```python
from build123d import *

# Parameters (mm, degrees)
BOSS_EXTRUDE1_DEPTH                     = 24
FILLET1_R                               = 1.5
SHELL1_T                                = -2
BOSS_EXTRUDE2_DEPTH                     = 6.2
CUT_EXTRUDE1_DEPTH                      = 5
FILLET2_R                               = 0.8
BOSS_EXTRUDE4_START                     = -1
SKETCH4_R                               = 5
BOSS_EXTRUDE4_DEPTH                     = 23
CBORE_FOR_M5_HEX_HEAD_BOLT1_D           = 3.7
CBORE_FOR_M5_HEX_HEAD_BOLT1_CBORE_D     = 7.5
CBORE_FOR_M5_HEX_HEAD_BOLT1_CBORE_DEPTH = 12


with BuildPart() as part:
    # Sketch1 → Boss-Extrude1 (new body)
    with BuildSketch(Plane(origin=(0, 0, 0), x_dir=(1, 0, 0), z_dir=(0, 1, 0))):
        with BuildLine():
            Line((74.5, -51.5), (74.5, 51.5))
            ThreePointArc((74.5, 51.5), (73.621320344, 53.621320344), (71.5, 54.5))
            Line((71.5, 54.5), (-71.5, 54.5))
            ThreePointArc((-71.5, 54.5), (-73.621320344, 53.621320344), (-74.5, 51.5))
            Line((-74.5, 51.5), (-74.5, -51.5))
            ThreePointArc((-74.5, -51.5), (-73.621320344, -53.621320344), (-71.5, -54.5))
            Line((-71.5, -54.5), (71.5, -54.5))
            ThreePointArc((71.5, -54.5), (73.621320344, -53.621320344), (74.5, -51.5))
        make_face()
    extrude(amount=BOSS_EXTRUDE1_DEPTH)

    # Fillet1
    fillet1_edges = [part.edges().sort_by_distance(p)[0] for p in [
        (-73.621320344, 24, -53.621320344),
        (-74.5, 24, 0),
        (-73.621320344, 24, 53.621320344),
        (0, 24, 54.5),
        (73.621320344, 24, 53.621320344),
        (74.5, 24, 0),
        (73.621320344, 24, -53.621320344),
        (0, 24, -54.5),
    ]]
    fillet(fillet1_edges, radius=FILLET1_R)

    # Shell1
    shell1_openings = [part.faces().sort_by_distance(p)[0] for p in [
        (0, 0, 0),
    ]]
    offset(amount=SHELL1_T, openings=shell1_openings, kind=Kind.INTERSECTION)

    # Sketch2 → Boss-Extrude2 (add)
    with BuildSketch(Plane(origin=(0, 0, 0), x_dir=(1, 0, 0), z_dir=(0, 1, 0))):
        with BuildLine():
            Line((-78, 51.5), (-78, -51.5))
            ThreePointArc((-78, -51.5), (-76.096194078, -56.096194078), (-71.5, -58))
            Line((-71.5, -58), (71.5, -58))
            ThreePointArc((71.5, -58), (76.096194078, -56.096194078), (78, -51.5))
            Line((78, -51.5), (78, 51.5))
            ThreePointArc((78, 51.5), (76.096194078, 56.096194078), (71.5, 58))
            Line((71.5, 58), (-71.5, 58))
            ThreePointArc((-71.5, 58), (-76.096194078, 56.096194078), (-78, 51.5))
        make_face()
        with BuildLine():
            Line((72.5, -51.5), (72.5, 51.5))
            ThreePointArc((72.5, 51.5), (72.207106781, 52.207106781), (71.5, 52.5))
            Line((71.5, 52.5), (-71.5, 52.5))
            ThreePointArc((-71.5, 52.5), (-72.207106781, 52.207106781), (-72.5, 51.5))
            Line((-72.5, 51.5), (-72.5, -51.5))
            ThreePointArc((-72.5, -51.5), (-72.207106781, -52.207106781), (-71.5, -52.5))
            Line((-71.5, -52.5), (71.5, -52.5))
            ThreePointArc((71.5, -52.5), (72.207106781, -52.207106781), (72.5, -51.5))
        make_face(mode=Mode.SUBTRACT)
    extrude(amount=BOSS_EXTRUDE2_DEPTH)

    # Sketch3 → Cut-Extrude1 (cut)
    with BuildSketch(Plane.XZ):
        with BuildLine():
            Line((-71.5, -56.5), (71.5, -56.5))
            ThreePointArc((71.5, -56.5), (75.035533906, -55.035533906), (76.5, -51.5))
            Line((76.5, -51.5), (76.5, 51.5))
            ThreePointArc((76.5, 51.5), (75.035533906, 55.035533906), (71.5, 56.5))
            Line((71.5, 56.5), (-71.5, 56.5))
            ThreePointArc((-71.5, 56.5), (-75.035533906, 55.035533906), (-76.5, 51.5))
            Line((-76.5, 51.5), (-76.5, -51.5))
            ThreePointArc((-76.5, -51.5), (-75.035533906, -55.035533906), (-71.5, -56.5))
        make_face()
        with BuildLine():
            Line((74, -51.5), (74, 51.5))
            ThreePointArc((74, 51.5), (73.267766953, 53.267766953), (71.5, 54))
            Line((71.5, 54), (-71.5, 54))
            ThreePointArc((-71.5, 54), (-73.267766953, 53.267766953), (-74, 51.5))
            Line((-74, 51.5), (-74, -51.5))
            ThreePointArc((-74, -51.5), (-73.267766953, -53.267766953), (-71.5, -54))
            Line((-71.5, -54), (71.5, -54))
            ThreePointArc((71.5, -54), (73.267766953, -53.267766953), (74, -51.5))
        make_face(mode=Mode.SUBTRACT)
    extrude(amount=-CUT_EXTRUDE1_DEPTH, mode=Mode.SUBTRACT)

    # Fillet2
    fillet2_edges = [part.edges().sort_by_distance(p)[0] for p in [
        (-76.096194078, 6.2, -56.096194078),
        (-78, 6.2, 0),
        (-76.096194078, 6.2, 56.096194078),
        (0, 6.2, 58),
        (76.096194078, 6.2, 56.096194078),
        (78, 6.2, 0),
        (76.096194078, 6.2, -56.096194078),
        (0, 6.2, -58),
        (74.5, 6.2, 0),
        (73.621320344, 6.2, -53.621320344),
        (0, 6.2, -54.5),
        (-73.621320344, 6.2, -53.621320344),
        (-74.5, 6.2, 0),
        (-73.621320344, 6.2, 53.621320344),
        (0, 6.2, 54.5),
        (73.621320344, 6.2, 53.621320344),
    ]]
    fillet(fillet2_edges, radius=FILLET2_R)

    # Sketch4 → Boss-Extrude4 (add)
    with BuildSketch(Plane(origin=(0, 24, 0), x_dir=(1, 0, 0), z_dir=(0, 1, 0)).offset(BOSS_EXTRUDE4_START)):
        with Locations((69, 49)):
            Circle(SKETCH4_R)
        with Locations((69, -49)):
            Circle(SKETCH4_R)
        with Locations((-69, 49)):
            Circle(SKETCH4_R)
        with Locations((-69, -49)):
            Circle(SKETCH4_R)
    extrude(amount=-BOSS_EXTRUDE4_DEPTH)

    # CBORE for M5 Hex Head Bolt1 (through all)
    with Locations(Plane(origin=(0, 24, 0), x_dir=(1, 0, 0), z_dir=(0, 1, 0))):
        with Locations((-69, -49), (69, -49), (-69, 49), (69, 49)):
            CounterBoreHole(CBORE_FOR_M5_HEX_HEAD_BOLT1_D / 2, CBORE_FOR_M5_HEX_HEAD_BOLT1_CBORE_D / 2, CBORE_FOR_M5_HEX_HEAD_BOLT1_CBORE_DEPTH)


solid = part.part
```
Geometry: final body of the model. Coordinates: model frame, mm. A direction names the side the tool comes from. Round coordinates to 2 decimals unless told otherwise and drop trailing zeros. Write each loop counter-clockwise with the first axis right and the second up, starting at its lowest first coordinate (ties: lowest second). Pieces come first, ordered by that corner, then holes. Notation, with made-up numbers: M -39,-2 L -17,-2 A5 ccw -17,2 Z; hole C 64,40.25 d10. An arc over 180 degrees is marked long. Answer in a Markdown table with one row per item. Add a question column.
(1) Draft query along X for faces 1 (the face through (-1, 15, 54.5)), 2 (the face through (72.464, 18.084, 50.436)). Return one class per face: pulls with the +X half, pulls with the -X half, needs draft (parallel to the pull), parting line crosses it, or undercut.
(2) Cut plane A-A, the plane y = 18.25. Return the cut outline in (x, z), then the cut area to 3 significant figures.
(3) Cut plane D-D, the plane z = -49. Give the number of separate pieces and of enclosed holes in the cut face, then the cut area to 3 significant figures.
(4) Cut plane C-C, the plane x = 61.5. Return the cut outline in (y, z), then the cut area to 3 significant figures.
(5) Reachability of faces 3 (the face through (-76.5, 2, 1)), 4 (the face through (70.468, 5.916, -47.874)), 5 (the face through (-65.536, 18.084, -47.564)) from +Z, -Z, +X, -X, +Y, -Y: full face, straight path, thin tool, end or side. Return the list, or none.
(6) Contact query for flat-ended pins moving along their axis: pin 1 (3 mm diameter, centred on y = 11.5, z = 29.5, fed in from +X); pin 2 (6 mm diameter, centred on y = 17.5, z = 8.5, fed in from -X); pin 3 (1 mm diameter, centred on x = 3, y = 8, fed in from -Z). Output: stop coordinate, or through.
(7) Ray query, L1, parallel to Z at x = -40.5, y = 1.5; L2, parallel to Z at x = -69, y = 7; L3, parallel to X at y = 16.5, z = 49. Return the intervals inside material, ascending.
(8) Cut plane B-B, the plane z = -26. Return the cut outline in (x, y).
Established:
| question | item | result |
|---|---|---|
| 1 | face 1 | needs draft |
| 1 | face 2 | undercut |
| 2 | outline | M -74.5,-51.5 A3 ccw -71.5,-54.5 L 71.5,-54.5 A3 ccw 74.5,-51.5 L 74.5,51.5 A3 ccw 71.5,54.5 L -71.5,54.5 A3 ccw -74.5,51.5 Z; hole C -69,-49 d7.5; hole C -69,49 d7.5; hole M -72.5,-45.43 A5 cw -65.43,-52.5 L 65.43,-52.5 A5 cw 72.5,-45.43 L 72.5,45.43 A5 cw 65.43,52.5 L -65.43,52.5 A5 cw -72.5,45.43 Z; hole C 69,-49 d7.5; hole C 69,49 d7.5 |
| 2 | area | 1,090 mm² |
| 3 | separate pieces | 3 |
| 3 | enclosed holes | 0 |
| 3 | area | 509 mm² |
| 4 | outline | M 0,-58 L 5.4,-58 A0.8 ccw 6.2,-57.2 L 6.2,-55.3 A0.8 cw 7,-54.5 L 22.5,-54.5 A1.5 ccw 24,-53 L 24,53 A1.5 ccw 22.5,54.5 L 7,54.5 A0.8 cw 6.2,55.3 L 6.2,57.2 A0.8 ccw 5.4,58 L 0,58 L 0,56.5 L 5,56.5 L 5,54 L 0,54 L 0,52.5 L 22,52.5 L 22,-52.5 L 0,-52.5 L 0,-54 L 5,-54 L 5,-56.5 L 0,-56.5 Z |
| 4 | area | 323 mm² |
| 5 | face 3 | -Y |
| 5 | face 4 | +Y, -Y |
| 5 | face 5 | +Y |
| 6 | pin 1 | x = 74.5 |
| 6 | pin 2 | x = -74.5 |
| 6 | pin 3 | z = -54.5 |
| 7 | L1 | -58 to -56.5, -54 to -52.5, 52.5 to 54, 56.5 to 58 |
| 7 | L2 | -54.5 to -50.85, -47.15 to -44, 44 to 47.15, 50.85 to 54.5 |
| 7 | L3 | -74.5 to -72.75, -65.25 to -64, 64 to 65.25, 72.75 to 74.5 |
| 8 | outline | M -78,0 L -76.5,0 L -76.5,5 L -74,5 L -74,0 L -72.5,0 L -72.5,22 L 72.5,22 L 72.5,0 L 74,0 L 74,5 L 76.5,5 L 76.5,0 L 78,0 L 78,5.4 A0.8 ccw 77.2,6.2 L 75.3,6.2 A0.8 cw 74.5,7 L 74.5,22.5 A1.5 ccw 73,24 L -73,24 A1.5 ccw -74.5,22.5 L -74.5,7 A0.8 cw -75.3,6.2 L -77.2,6.2 A0.8 ccw -78,5.4 Z |
